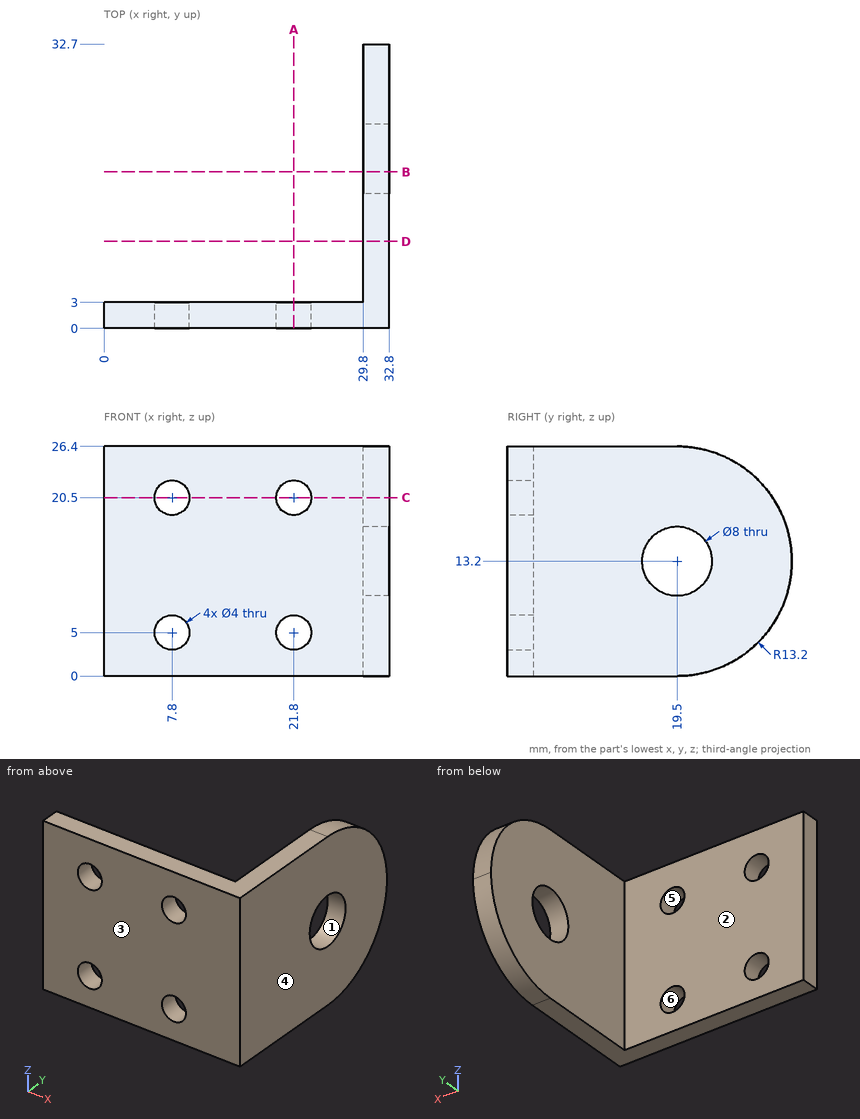
Design review of the part shown in the three views and the two pictorial views. Dimensions are in mm from the part's minimum x, y and z. A direction names the side the tool comes from. Round coordinates to 2 decimals unless told otherwise and drop trailing zeros. Write each loop counter-clockwise with the first axis right and the second up, starting at its lowest first coordinate (ties: lowest second). Pieces come first, ordered by that corner, then holes. Notation, with made-up numbers: (83.5, -21.5) -> (113.5, -21.5) arc R21 ccw to (113.5, 9.5) -> close; hole circle Ø8 at (68, -32). An arc over 180 degrees is marked (long way). One line per question, with ' | ' between items. Start each with the question number.
1) Mouldability with a two-part tool opening along X and no side actions: class the marked faces 3, 4, 5 and 6 as +X half, -X half, draft (parallel to the pull), parting line (faces both ways), or undercut.
2) Wall thickness on line 1 along X through (y, z) = (2.15, 20.5); line 2 along Z through (x, y) = (21, 1); line 3 along X through (y, z) = (14, 23.25): over which ranges is each line inside the solid? List them lowest first.
3) Add section D-D (y = 10). Write out the cut boundary in (x, z), and give its area (3 significant figures).
4) Machinability: for the marked faces 1 and 2, which of the approach directions +Z, -Z, +X, -X, +Y, -Y give a long, thin tool a straight path to every point of the face, cutting with its end or side? Answer none if there is none.
5) Add section C-C (z = 20.5). Write out the cut boundary in (x, y), and give its area (3 significant figures).
6) Add section B-B (y = 18). Write out the cut boundary in (x, z).
7) For pin 1 Ø13 at (x, z) = (19, 18) entering from +Y; pin 2 Ø8 at (y, z) = (11.5, 13) entering from -X, all flat-tipped, find the tip position at first contact; note any pin that passes through.
8) Add section A-A (x = 21.8). Write out the cut boundary in (y, z).
Reported:
1) face 3: draft | face 4: +X half | face 5: undercut | face 6: undercut
2) line 1: x = 0 to 5.8, 9.8 to 19.8, 23.8 to 32.8 | line 2: z = 0 to 3.17, 6.83 to 18.67, 22.33 to 26.4 | line 3: x = 29.8 to 32.8
3) outline: (29.8, 0) -> (32.8, 0) -> (32.8, 26.4) -> (29.8, 26.4) -> close | area: 79.2 mm²
4) face 1: +X, -X | face 2: +Z, -Z, -X, +Y
5) outline: (0, 0) -> (5.8, 0) -> (5.8, 3) -> (0, 3) -> close; (9.8, 0) -> (19.8, 0) -> (19.8, 3) -> (9.8, 3) -> close; (23.8, 0) -> (32.8, 0) -> (32.8, 30.5) -> (29.8, 30.5) -> (29.8, 3) -> (23.8, 3) -> close | area: 157 mm²
6) outline: (29.8, 0) -> (32.8, 0) -> (32.8, 9.49) -> (29.8, 9.49) -> close; (29.8, 16.91) -> (32.8, 16.91) -> (32.8, 26.4) -> (29.8, 26.4) -> close
7) pin 1: stops at y = 3 | pin 2: stops at x = 29.8
8) outline: (0, 0) -> (3, 0) -> (3, 3) -> (0, 3) -> close; (0, 7) -> (3, 7) -> (3, 18.5) -> (0, 18.5) -> close; (0, 22.5) -> (3, 22.5) -> (3, 26.4) -> (0, 26.4) -> close
